from build123d import *

# Parameters (mm, degrees)
BOSS_EXTRUDE1_DEPTH        = 80
BOSS_EXTRUDE3_DEPTH        = 8.5
BOSS_EXTRUDE4_START        = -8.5
BOSS_EXTRUDE4_DEPTH        = 8.5
F_10_0_10_DIAMETER_HOLE1_D = 10
CUT_EXTRUDE1_DEPTH         = 133.249763765


with BuildPart() as part:
    # Sketch2 → Boss-Extrude1 (new body)
    with BuildSketch(Plane.XY):
        with BuildLine():
            Line((-21, -37.5), (0, -37.5))
            Line((0, -37.5), (0, -17.5))
            ThreePointArc((0, -17.5), (-15.231429157, -8.617050879), (-15, 9.013878189))
            ThreePointArc((-15, 9.013878189), (-11.342217923, 13.326818547), (-6.5, 16.248076809))
            Line((-6.5, 16.248076809), (-6.5, 34.391132578))
            ThreePointArc((-6.5, 34.391132578), (-26.949025956, 22.332711434), (-35, 0))
            Line((-35, 0), (-35, -28))
            Line((-35, -28), (-53, -28))
            Line((-53, -28), (-53, -44))
            Line((-53, -44), (-21, -44))
            Line((-21, -44), (-21, -37.5))
        make_face()
        with BuildLine():
            Line((0, -17.5), (0, -37.5))
            Line((0, -37.5), (21, -37.5))
            Line((21, -37.5), (21, -44))
            Line((21, -44), (53, -44))
            Line((53, -44), (53, -28))
            Line((53, -28), (35, -28))
            Line((35, -28), (35, 0))
            ThreePointArc((35, 0), (26.949025956, 22.332711434), (6.5, 34.391132578))
            Line((6.5, 34.391132578), (6.5, 16.248076809))
            ThreePointArc((6.5, 16.248076809), (11.342217923, 13.326818547), (15, 9.013878189))
            ThreePointArc((15, 9.013878189), (15.231429157, -8.617050879), (0, -17.5))
        make_face()
    extrude(amount=BOSS_EXTRUDE1_DEPTH)

    # Sketch5 → Boss-Extrude3 (add)
    with BuildSketch(Plane.ZY.offset(-6.5)):
        with BuildLine():
            Line((27, 34.391132578), (27, 50))
            ThreePointArc((27, 50), (40, 63), (53, 50))
            Line((53, 50), (53, 34.391132578))
            ThreePointArc((53, 34.391132578), (40, 21.391132578), (27, 34.391132578))
        make_face()
    extrude(amount=-BOSS_EXTRUDE3_DEPTH)

    # Sketch3 → Boss-Extrude4 (add)
    with BuildSketch(Plane(origin=(-6.5, 0, 0), x_dir=(0, 0, -1), z_dir=(1, 0, 0)).offset(BOSS_EXTRUDE4_START)):
        with BuildLine():
            Line((-53, 34.391132578), (-53, 50))
            ThreePointArc((-53, 50), (-40, 63), (-27, 50))
            Line((-27, 50), (-27, 34.391132578))
            ThreePointArc((-27, 34.391132578), (-40, 21.391132578), (-53, 34.391132578))
        make_face()
    extrude(amount=BOSS_EXTRUDE4_DEPTH)

    # Ø10.0 (10) Diameter Hole1 (through all)
    with Locations(Plane(origin=(15, 50, 40), x_dir=(0, 1, 0), z_dir=(1, 0, 0))):
        with Locations((0, 0)):
            Hole(F_10_0_10_DIAMETER_HOLE1_D / 2)

    # Sketch7 → Cut-Extrude1 (cut, through all)
    with BuildSketch(Plane(origin=(0, -28, 0), x_dir=(1, 0, 0), z_dir=(0, 1, 0))):
        with BuildLine():
            Line((-40, -12.5), (-40, -67.5))
            ThreePointArc((-40, -67.5), (-44, -71.5), (-48, -67.5))
            Line((-48, -67.5), (-48, -12.5))
            ThreePointArc((-48, -12.5), (-44, -8.5), (-40, -12.5))
        make_face()
        with BuildLine():
            Line((40, -12.5), (40, -67.5))
            ThreePointArc((40, -67.5), (44, -71.5), (48, -67.5))
            Line((48, -67.5), (48, -12.5))
            ThreePointArc((48, -12.5), (44, -8.5), (40, -12.5))
        make_face()
    extrude(amount=-CUT_EXTRUDE1_DEPTH, mode=Mode.SUBTRACT)


solid = part.part
The listing builds one solid part. Answer for the finished solid, in the listing's coordinates (mm). A direction names the side the tool comes from. Coordinates: 2 decimals unless noted, no trailing zeros. Order: outer loops, then holes, each group sorted by start corner. A loop starts at its lowest first (then second) coordinate and runs counter-clockwise, first axis right, second up.
Q1. A cutting plane is placed at B-B, the plane x = 44. Write down the section's boundary in (y, z).
Q2. Consider line 1 (X direction, y = 1, z = 58); line 2 (Z direction, x = 8.75, y = 50); line 3 (X direction, y = -38, z = 3). Determine where each line is inside the solid, lowest interval first.
Q3. A cutting plane is placed at C-C, the plane y = -29.5. Write down the section's boundary in (x, z).
Q4. Given P1, Ø9, axis at x = 43.5, z = 22, coming from the +Y side; P2, Ø4, axis at x = 10.5, y = 45.5, coming from the +Z side; P3, Ø4, axis at y = 16, z = 54, coming from the +X side; P4, Ø8, axis at y = 50, z = 40, coming from the -X side, each flat-ended and moving along its own axis, determine where each tip first touches the part or whether it passes through.
Q5. For a pull along Y with two mould halves and no side action, classify faces 4 (the face through (-34, -44, 39)), 5 (the face through (43.9, -35.9, 71.5)), 6 (the face through (-12.7, 33.64, 27.02)) as pulls with the +Y half, pulls with the -Y half, needs draft (parallel to the pull), parting line crosses it, or undercut.
Q6. A cutting plane is placed at A-A, the plane y = -10.5. Write down the section's boundary in (x, z).
Q7. Which of the six approach directions +Z, -Z, +X, -X, +Y, -Y give full straight-line access (tool end or side, diameter ignored) to faces 1 (the face through (-48, -36, 40)), 2 (the face through (11, 42, 53)), 3 (the face through (50, -28, 39))?
Q8. A cutting plane is placed at D-D, the plane z = 48.5. Write down the section's boundary in (x, y).
Answers follow:
1. outline: (-44, 0) - (-28, 0) - (-28, 8.5) - (-44, 8.5) - close; (-44, 71.5) - (-28, 71.5) - (-28, 80) - (-44, 80) - close
2. line 1: x = -34.99 to -17.47, 17.47 to 34.99
2. line 2: z = 27 to 35, 45 to 53
2. line 3: x = -53 to -21, 21 to 53
3. outline: (-53, 0) - (53, 0) - (53, 80) - (-53, 80) - close; hole (-48, 12.5) arc R4 ccw to (-40, 12.5) - (-40, 67.5) arc R4 ccw to (-48, 67.5) - close; hole (40, 12.5) arc R4 ccw to (48, 12.5) - (48, 67.5) arc R4 ccw to (40, 67.5) - close
4. P1: stops at y = -28
4. P2: stops at z = 53
4. P3: stops at x = 32.08
4. P4: passes through
5. face 4: pulls with the -Y half
5. face 5: needs draft
5. face 6: undercut
6. outline: (-35, 0) - (-14, 0) - (-14, 80) - (-35, 80) - close; (14, 0) - (35, 0) - (35, 80) - (14, 80) - close
7. face 1: +Y, -Y
7. face 2: +Z, +X, -X, +Y
7. face 3: +Z, -Z, +X, +Y
8. outline: (-53, -44) - (-48, -44) - (-48, -28) - (-53, -28) - close; (-40, -44) - (-21, -44) - (-21, -37.5) - (21, -37.5) - (21, -44) - (40, -44) - (40, -28) - (35, -28) - (35, 0) arc R35 ccw to (15, 31.62) - (15, 59.84) - (6.5, 59.84) - (6.5, 16.25) arc R17.5 cw (long way) to (-6.5, 16.25) - (-6.5, 59.84) - (-15, 59.84) - (-15, 31.62) arc R35 ccw to (-35, 0) - (-35, -28) - (-40, -28) - close; (48, -44) - (53, -44) - (53, -28) - (48, -28) - close
